Work out the finished part from the listing and answer in its coordinate system (mm). A direction names the side the tool comes from. Round coordinates to 2 decimals unless told otherwise and drop trailing zeros. Write each loop counter-clockwise with the first axis right and the second up, starting at its lowest first coordinate (ties: lowest second). Pieces come first, ordered by that corner, then holes. Notation, with made-up numbers: M 73.25,58 L 122.25,58 A25 ccw 122.25,72 Z; hole C 77,32.5 d5. An arc over 180 degrees is marked long. Answer in a Markdown table with one row per item.
```python
from build123d import *

# Parameters (mm, degrees)
F1_DEPTH = 88.9
F2_W     = 38.1
F2_H     = 50.8
F3_DEPTH = 38.1


with BuildPart() as f1:
    # F0 (on Right) → F1 (new body)
    with BuildSketch(Plane.YZ):
        Polygon((-10.972409, 35.849495), (-74.472409, 35.849495), (-74.472409, 10.449495), (-36.372409, 10.449495), (-36.372409, -40.350505), (39.827591, -40.350505), (39.827591, -14.950505), (-10.972409, -14.950505), align=None)
    extrude(amount=-F1_DEPTH)

    # F2 (on face) → F3 (join)
    with BuildSketch(Plane(origin=(-88.9, 0, 0), x_dir=(0, -1, 0), z_dir=(-1, 0, 0))):
        with Locations((-8.077591, 10.449495)):
            Rectangle(F2_W, F2_H)
    extrude(amount=-F3_DEPTH)


solid = f1.part
```
1. The part is cut by section B-B (z = 23). Determine the outline of the cut face in (x, y).
Calculated:
| item | result |
|---|---|
| outline | M -88.9,-74.47 L 0,-74.47 L 0,-10.97 L -50.8,-10.97 L -50.8,27.13 L -88.9,27.13 Z |
2. Consider line 1 along Y through (x, z) = (-67, 18.5); line 2 along Y through (x, z) = (-57.5, 7); line 3 along X through (y, z) = (-7, 15). Determine where each line is inside the solid, lowest interval first. Write a range as from..to.
Calculated:
| item | result |
|---|---|
| line 1 | y = -74.47..27.13 |
| line 2 | y = -36.37..27.13 |
| line 3 | x = -88.9..-50.8 |
3. The part is cut by section A-A (x = -15). Determine the outline of the cut face in (y, z), plus the area to 3 significant figures.
Calculated:
| item | result |
|---|---|
| outline | M -74.47,10.45 L -36.37,10.45 L -36.37,-40.35 L 39.83,-40.35 L 39.83,-14.95 L -10.97,-14.95 L -10.97,35.85 L -74.47,35.85 Z |
| area | 4,190 mm² |
4. Given pin 1 (6 mm diameter, centred on x = -63, z = -13.5, fed in from -Y); pin 2 (15 mm diameter, centred on x = -25.5, y = 14, fed in from +Z); pin 3 (12 mm diameter, centred on y = -7, z = -29, fed in from +X); pin 4 (19 mm diameter, centred on y = 1.5, z = 7, fed in from +X), each flat-ended and moving along its own axis, determine where each tip first touches the part or whether it passes through.
Calculated:
| item | result |
|---|---|
| pin 1 | stops at y = -36.37 |
| pin 2 | stops at z = -14.95 |
| pin 3 | stops at x = 0 |
| pin 4 | stops at x = -50.8 |
5. The part is cut by section D-D (x = -69.5). Determine the outline of the cut face in (y, z), plus the area to 3 significant figures.
Calculated:
| item | result |
|---|---|
| outline | M -74.47,10.45 L -36.37,10.45 L -36.37,-40.35 L 39.83,-40.35 L 39.83,-14.95 L 27.13,-14.95 L 27.13,35.85 L -74.47,35.85 Z |
| area | 6,130 mm² |
6. A tool of negligible diameter and unlimited length cuts with its end or side. For faces 1 (the flat face through (-70, 27.128, 10)), 2 (the flat face through (-25, -10.972, 10)), 3 (the flat face through (-44, -36.372, -15)), from which of +Z, -Z, +X, -X, +Y, -Y can it reach the whole face along a straight path? Write none if from no direction.
Calculated:
| item | result |
|---|---|
| face 1 | +Z, +X, -X, +Y |
| face 2 | +Z, +X, +Y |
| face 3 | -Z, +X, -X, -Y |
7. The part is cut by section C-C (y = 25.5). Determine the outline of the cut face in (x, z), plus the area to 3 significant figures.
Calculated:
| item | result |
|---|---|
| outline | M -88.9,-40.35 L 0,-40.35 L 0,-14.95 L -50.8,-14.95 L -50.8,35.85 L -88.9,35.85 Z |
| area | 4,190 mm² |
